from build123d import *

# Parameters (mm, degrees)
F0_R     = 2.5
F1_DEPTH = 6


with BuildPart() as f1:
    # F0 (on Top) → F1 (new body)
    with BuildSketch(Plane.XY):
        with BuildLine():
            ThreePointArc((60, 120), (21.961524, 81.961524), (8.038476, 30))
            ThreePointArc((8.038476, 30), (60, 16.076952), (111.961524, 30))
            ThreePointArc((111.961524, 30), (98.038476, 81.961524), (60, 120))
        make_face()
        with Locations((56, 56)):
            Circle(F0_R, mode=Mode.SUBTRACT)
        with Locations((56, 64)):
            Circle(F0_R, mode=Mode.SUBTRACT)
        with BuildLine():
            Line((35.802732, 41.410898), (53.592414, 51.681776))
            ThreePointArc((53.592414, 51.681776), (60, 49.5), (66.407586, 51.681776))
            Line((66.407586, 51.681776), (84.197268, 41.410898))
            Line((84.197268, 41.410898), (99.174061, 32.764043))
            ThreePointArc((99.174061, 32.764043), (60, 23.39746), (20.825939, 32.764043))
            Line((20.825939, 32.764043), (35.802732, 41.410898))
        make_face(mode=Mode.SUBTRACT)
        with Locations((64, 56)):
            Circle(F0_R, mode=Mode.SUBTRACT)
        with Locations((64, 64)):
            Circle(F0_R, mode=Mode.SUBTRACT)
        with BuildLine():
            ThreePointArc((16.825939, 39.692247), (28.30127, 78.30127), (56, 107.54371))
            Line((56, 107.54371), (56, 85))
            Line((56, 85), (56, 69.708244))
            ThreePointArc((56, 69.708244), (50.906733, 65.25), (49.592414, 58.60998))
            Line((49.592414, 58.60998), (31.802732, 48.339102))
            Line((31.802732, 48.339102), (16.825939, 39.692247))
        make_face(mode=Mode.SUBTRACT)
        with BuildLine():
            ThreePointArc((64, 107.54371), (91.69873, 78.30127), (103.174061, 39.692247))
            Line((103.174061, 39.692247), (88.197268, 48.339102))
            Line((88.197268, 48.339102), (70.407586, 58.60998))
            ThreePointArc((70.407586, 58.60998), (69.093267, 65.25), (64, 69.708244))
            Line((64, 69.708244), (64, 85))
            Line((64, 85), (64, 107.54371))
        make_face(mode=Mode.SUBTRACT)
    extrude(amount=F1_DEPTH)


solid = f1.part
Geometry: final body of the model. Coordinates: model frame, mm. A direction names the side the tool comes from. Coordinates: 2 decimals unless noted, no trailing zeros. Loops run counter-clockwise (first coordinate to the right, second up) from the corner with the lowest first, then second, coordinate; pieces in that order, holes last. Notation, with made-up numbers: M 38.5,-37.75 L 58.5,-37.75 A25 cw 58.5,-15.75 Z; hole C 6.5,62 d5. An arc over 180 degrees is marked long. One line per item, written item: value. Start each with the question number.
1) Pin query (flat end, axial travel): P1, Ø3, axis at x = 76.5, z = 2.5, coming from the -Y side; P2, Ø1.8, axis at y = 81.5, z = 1.5, coming from the +X side; P3, Ø4.5, axis at x = 64, y = 56, coming from the +Z side (3 decimals); P4, Ø2, axis at y = 77.5, z = 4.5, coming from the -X side. Return the tip coordinate at first contact, or that it passes through.
2) Cut plane D-D (y = 64). Return loops of the section in (x, z).
3) Cut plane B-B (y = 80). Return loops of the section in (x, z), then the cut area to 3 significant figures.
4) Cut plane A-A (z = 1.9). Return loops of the section in (x, y), then the cut area to 3 significant figures.
5) Draft query along Y for faces 3 (the cylindrical face through (66.385, 64.751, 2.958)), 4 (the cylindrical face through (22.345, 82.62, 2.958)), 5 (the cylindrical face through (50.955, 65.333, 2.958)), 6 (the cylindrical face through (59.24, 16.08, 2.96)). Return one class per face: released by +Y, released by -Y, zero draft, split by the parting line, or undercut.
6) Reachability of faces 1 (the flat face through (56, 89, 3)), 2 (the flat face through (60, 57, 0)) from +Z, -Z, +X, -X, +Y, -Y: full face, straight path, thin tool, end or side. Return the list, or none.
7) Material intervals for L1, parallel to X at y = 80.5, z = 3.65; L2, parallel to Y at x = 88, z = 2.05; L3, parallel to Y at x = 46, z = 2.55, sorted ascending. Write a range as from..to.
8) Cut plane C-C (x = 22.5). Return loops of the section in (y, z).
Evaluation:
1. P1: y = 17.17
1. P2: x = 98.81
1. P3: through
1. P4: x = 19.02
2. outline: M 13.76,0 L 21.7,0 L 21.7,6 L 13.76,6 Z; M 50.29,0 L 53.5,0 L 53.5,6 L 50.29,6 Z; M 58.5,0 L 61.5,0 L 61.5,6 L 58.5,6 Z; M 66.5,0 L 69.71,0 L 69.71,6 L 66.5,6 Z; M 98.3,0 L 106.24,0 L 106.24,6 L 98.3,6 Z
3. outline: M 20.86,0 L 29.31,0 L 29.31,6 L 20.86,6 Z; M 56,0 L 64,0 L 64,6 L 56,6 Z; M 90.69,0 L 99.14,0 L 99.14,6 L 90.69,6 Z
3. area: 149 mm^2
4. outline: M 8.04,30 A103.92 ccw 111.96,30 A103.92 ccw 60,120 A103.92 ccw Z; hole M 16.83,39.69 L 49.59,58.61 A10.5 cw 56,69.71 L 56,107.54 A86.6 ccw Z; hole M 20.83,32.76 A86.6 ccw 99.17,32.76 L 66.41,51.68 A10.5 cw 53.59,51.68 Z; hole C 56,56 d5; hole C 56,64 d5; hole C 64,56 d5; hole C 64,64 d5; hole M 64,69.71 A10.5 cw 70.41,58.61 L 103.17,39.69 A86.6 ccw 64,107.54 Z
4. area: 3,520 mm^2
5. face 3: undercut
5. face 4: released by +Y
5. face 5: undercut
5. face 6: released by -Y
6. face 1: +Z, -Z
6. face 2: -Z, +X, -X, +Y, -Y
7. L1: 21.13..29.61, 56..64, 90.39..98.87
7. L2: 19.92..28.05, 39.22..48.45, 84.15..96.38
7. L3: 17.02..24.54, 47.3..56.54, 99.94..110.31
8. outline: M 23.08,0 L 31.94,0 L 31.94,6 L 23.08,6 Z; M 33.73,0 L 42.97,0 L 42.97,6 L 33.73,6 Z; M 66.16,0 L 82.88,0 L 82.88,6 L 66.16,6 Z
